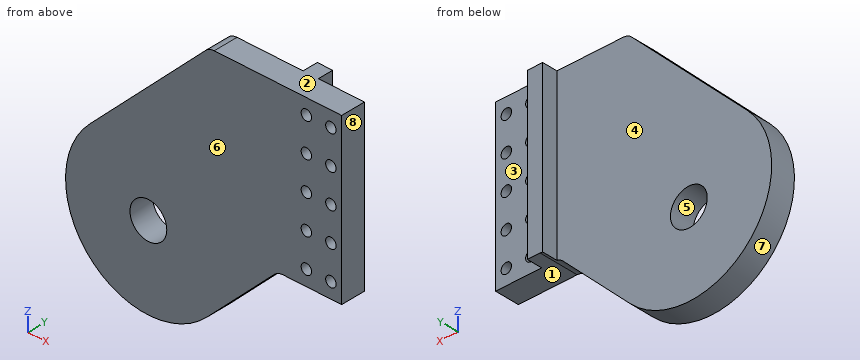
Autodesk Inventor part; units mm, degrees
ref_plane "YZ Plane" through (0, 0, 0) normal (1, 0, 0) x (0, 1, 0)
ref_plane "XZ Plane" through (0, 0, 0) normal (0, 1, 0) x (-1, 0, 0)
ref_plane "XY Plane" through (0, 0, 0) normal (0, 0, 1) x (1, 0, 0)
sketch "Skizze1" plane through (0, 0, 0) normal (0, 1, 0) x (-1, 0, 0)
  line L0 (20.8162, -27) -> (0, -27)
  line L1 (0, -27) -> (0, 27)
  line L2 (20.8162, -27) -> (43.9081, -50.0919)
  arc A0 (43.9081, -50.0919) -> (82.0919, -11.9081) centre (63, -31) ccw
  line L3 (82.0919, -11.9081) -> (43.1838, 27)
  line L4 (0, 27) -> (43.1838, 27)
  point P0 (0, 0)
  dimension "d0" = 54
  dimension "d40" = 135
  dimension "d42" = 54
  dimension "d43" = 31
  dimension "d47" = 63
extrude "Extrusion1" add sketch "Skizze1" along normal blind 8
sketch "Skizze3" plane through (0, 8, 0) normal (0, 1, 0) x (1, 0, 0)
  line L0 (0, 0) -> (-17.1865, 0) construction
  line L1 (0, -27) -> (0, 27) construction
  line L2 (0, -27) -> (0, 27) construction
  line L3 (0, 27) -> (-20.8162, 27) construction
  line L4 (-18, -27) -> (0, -27) construction
  line L5 (0, 27) -> (-20.8162, 27) construction
  line L6 (-20.8162, 27) -> (-43.9081, 50.0919)
  arc A0 (-43.9081, 50.0919) -> (-82.0919, 11.9081) centre (-63, 31) ccw
  line L7 (-82.0919, 11.9081) -> (-43.1838, -27)
  line L8 (-43.1838, -27) -> (0, -27)
  arc A1 (-43.9081, 50.0919) -> (-82.0919, 11.9081) centre (-63, 31) ccw
  circle A2 centre (-63, 31) radius 6
  point P0 (-18, 27)
  dimension "d48" = 12
extrude "Extrusion3" [suppressed]
sketch "Skizze5" plane through (0, 8, 0) normal (0, 1, 0) x (1, 0, 0)
  line L0 (0, -27) -> (0, 27)
  line L1 (0, 27) -> (-20.8162, 27)
  line L2 (-15, -27) -> (-20, -27)
  line L3 (-20, -27) -> (-20, 27)
  line L4 (-20, 27) -> (-15, 27)
  line L5 (-15, 27) -> (-15, -27)
  line L6 (-82.0919, 11.9081) -> (-43.1838, -27)
  line L7 (-43.1838, -27) -> (0, -27)
  line L8 (-20.8162, 27) -> (-43.9081, 50.0919)
  arc A0 (-43.9081, 50.0919) -> (-82.0919, 11.9081) centre (-63, 31) ccw
  point P0 (0, 0)
  dimension "d14" = 15
  dimension "d15" = 5
extrude "Extrusion4" add sketch "Skizze5" along normal blind 5 contours L2 L3 L1 L5
sketch "Skizze6" plane through (0, 8, 0) normal (0, 1, 0) x (1, 0, 0)
  line L0 (-15, 27) -> (-15, -27)
  line L1 (0, -27) -> (0, 27)
  line L2 (0, 27) -> (-15, 27)
  line L3 (0, 0) -> (67.4565, 0) construction
  line L4 (-15, -27) -> (0, -27)
  point P0 (-3.5, 0)
  dimension "d18" = 3.5
hole "Bohrung1" at (-3.5, 8, 0) direction (0, -1, 0) diameter 3.4 end through all
pattern_linear "Rechteckige Anordnung1" count 5 spacing 11 along (0, 0, -1) count 2 spacing 8 along (-1, 0, 0) of "Bohrung1" first direction both ways yes
sketch "Skizze7" plane through (0, 0, 0) normal (0, -1, 0) x (1, 0, 0)
  circle A0 centre (-63, -31) radius 6
  circle A1 centre (-63, -31) radius 10 construction
  line L0 (-63, -45.6355) -> (-63, -17.0341)
  line L1 (-76.3383, -31) -> (-50.0008, -31)
  circle A2 centre (-63, -31) radius 6
  point P0 (0, 0)
  point P1 (-63, -41)
  point P2 (-73, -31)
  point P3 (-63, -21)
  point P4 (-53, -31)
  dimension "d32" = 20
hole "Bohrung2" [suppressed]
fillet "Rundung1" radius 4 2 edges at (-20.8162, 4, -27) (-43.1838, 4, 27)
sketch "Skizze8" plane through (0, 8, 0) normal (0, 1, 0) x (1, 0, 0)
  arc A0 (-43.9081, 50.0919) -> (-82.0919, 11.9081) centre (-63, 31) ccw
  circle A1 centre (-63, 31) radius 6
  circle A2 centre (-63, 31) radius 4
  point P0 (0, 0)
  dimension "d50" = 12
  dimension "d51" = 8
extrude "Extrusion5" add sketch "Skizze8" along normal blind 3 contours A1 | A2
extrude "Extrusion6" add sketch "Skizze8" along normal blind 10 contours A2
sketch "Skizze9" plane through (0, 0, 0) normal (0, -1, 0) x (1, 0, 0)
  circle A0 centre (-63, -31) radius 4
  circle A1 centre (-63, -31) radius 6
  point P0 (0, 0)
extrude "Extrusion7" cut sketch "Skizze9" against normal through all contours A0 | A1
equation "\"d42\" = d0"
properties part number "dynamixel_pro_frame_part2" material "Aluminium 6061"
Build history of the part. All positions in model axes, mm. Face numbers are marked on the shaded views. A direction names the side the tool comes from. Round coordinates to 2 decimals unless told otherwise and drop trailing zeros. Loops run counter-clockwise (first coordinate to the right, second up) from the corner with the lowest first, then second, coordinate; pieces in that order, holes last. Notation, with made-up numbers: M 21.5,78 L 42.5,78 A22 cw 42.5,100 Z; hole C 84,60.5 d7. An arc over 180 degrees is marked long. Answer as CSV lines item,"result".
1. Cut at C-C on z = 0. Write the cut outline in (x, y), then the cut area to 3 significant figures.
Resolved:
outline,"M -70.18,0 L -13.2,0 L -13.2,8 L -15,8 L -15,13 L -20,13 L -20,8 L -70.18,8 Z; M -9.8,0 L -5.2,0 L -5.2,8 L -9.8,8 Z; M -1.8,0 L 0,0 L 0,8 L -1.8,8 Z"
area,"532 mm²"
2. Cut at B-B on x = -3.5. Write the cut outline in (y, z).
Resolved:
outline,"M 0,-27 L 8,-27 L 8,-23.7 L 0,-23.7 Z; M 0,-20.3 L 8,-20.3 L 8,-12.7 L 0,-12.7 Z; M 0,-9.3 L 8,-9.3 L 8,-1.7 L 0,-1.7 Z; M 0,1.7 L 8,1.7 L 8,9.3 L 0,9.3 Z; M 0,12.7 L 8,12.7 L 8,20.3 L 0,20.3 Z; M 0,23.7 L 8,23.7 L 8,27 L 0,27 Z"
3. Wall check: probe 1 along Z at (x, y) = (-3.5, 4); probe 2 along X at (y, z) = (3.5, 10); probe 3 along X at (y, z) = (4.5, -0.5). Give the ranges that are in metal, low to high. Write a range as [from, to].
Resolved:
probe 1,"z = [-27, -23.7], [-20.3, -12.7], [-9.3, -1.7], [1.7, 9.3], [12.7, 20.3], [23.7, 27]"
probe 2,"x = [-60.18, -12.87], [-10.13, -4.87], [-2.13, 0]"
probe 3,"x = [-70.68, -13.12], [-9.88, -5.12], [-1.88, 0]"
4. Cut at D-D on x = -63. Write the cut outline in (y, z), then the cut area to 3 significant figures.
Resolved:
outline,"M 0,-58 L 8,-58 L 8,-37 L 0,-37 Z; M 0,-25 L 8,-25 L 8,7.18 L 0,7.18 Z"
area,"425 mm²"
5. Two-plate mould, pull along X, no slides. Class the marked faces 5, 6, 7 and 8: released by +X, released by -X, zero draft, split by the parting line, or undercut.
Resolved:
face 5,"undercut"
face 6,"zero draft"
face 7,"split by the parting line"
face 8,"released by +X"
6. Flat gauge pins, fed straight in: P1, Ø4, axis at y = 11.5, z = 13, coming from the -X side; P2, Ø4, axis at y = 8.5, z = -21, coming from the -X side; P3, Ø1, axis at y = 9, z = -28.5, coming from the -X side; P4, Ø6, axis at x = -50, y = 5.5, coming from the -Z side. Where does each tip first touch, or does it go through?
Resolved:
P1,"stops at x = -20"
P2,"stops at x = -88.77"
P3,"passes through"
P4,"stops at z = -56.08"
7. 3-axis set-ups, long thin cutter, end or side, ignore diameter. For the marked faces 1, 2, 3 and 4: which of +Z, -Z, +X, -X, +Y, -Y reach the whole face in a straight line?
Resolved:
face 1,"-Z, +X, +Y, -Y"
face 2,"+Z, +X, -X, +Y, -Y"
face 3,"+Z, -Z, +X, +Y"
face 4,"+Z, -Z, -X, +Y"
8. Cut at A-A on y = 7. Count the separate pieces of the cut face and the enclosed holes in it, then the cut area to 3 significant figures.
Resolved:
separate pieces,"1"
enclosed holes,"11"
area,"5,040 mm²"
